Work out the finished part from the listing and answer in its coordinate system (mm). Coordinates: 2 decimals unless noted, no trailing zeros. Write each loop counter-clockwise with the first axis right and the second up, starting at its lowest first coordinate (ties: lowest second). Pieces come first, ordered by that corner, then holes. Notation, with made-up numbers: (9, -8.5) -> (13, -8.5) arc R4 ccw to (13, -2.5) -> close; hole circle Ø8 at (-34, 89.25). An arc over 180 degrees is marked (long way). Write each question's results on one line, items separated by ' | '. Start each with the question number.
Autodesk Inventor part; units mm, degrees
ref_plane "YZ Plane" through (0, 0, 0) normal (1, 0, 0) x (0, 1, 0)
ref_plane "XZ Plane" through (0, 0, 0) normal (0, 1, 0) x (-1, 0, 0)
ref_plane "XY Plane" through (0, 0, 0) normal (0, 0, 1) x (1, 0, 0)
sketch "スケッチ1" plane through (0, 0, 0) normal (0, 0, 1) x (1, 0, 0)
  circle A0 centre (0, 0) radius 8
  circle A1 centre (0, 0) radius 12
  dimension "d0" = 16
  dimension "d1" = 24
extrude "押し出し1" add sketch "スケッチ1" along normal blind 1
sketch "スケッチ2" plane through (0, 0, 1) normal (0, 0, 1) x (1, 0, 0)
  circle A0 centre (0, 0) radius 9
  circle A1 centre (0, 0) radius 12
  circle A2 centre (0, 0) radius 8
  dimension "d4" = 18
extrude "押し出し2" add sketch "スケッチ2" along normal blind 7 contours A0
chamfer "面取り1" distance 0.5 angle 45 1 edges at (-9, 0, 8)
properties part number "オイレスw10f16-18a" material "アセタール樹脂、黒"
1. Given pin 1 Ø1.5 at (x, z) = (5, 6.5) entering from -Y; pin 2 Ø3 at (y, z) = (-7.5, 6.5) entering from -X, each flat-ended and moving along its own axis, determine where each tip first touches the part or whether it passes through.
2. Find section A-A on x = 0. Give the vertices of the cut face in (y, z).
3. Find the intervals of material crossed by L1, parallel to Y at x = 0, z = 3.5; L2, parallel to Z at x = 1, y = -9.25; L3, parallel to Y at x = 3.25, z = 2.25, in increasing order.
4. Find section C-C on z = 2.5. Give the vertices of the cut face in (x, y).
5. Determine the mould class of faces 1 (the face through (2, 9, 1)), 2 (the face through (-1.73, 7.81, 3.94)), 3 (the face through (-1.172, -8.923, 4.204)) for opening direction Y: pulls with the +Y half, pulls with the -Y half, needs draft (parallel to the pull), parting line crosses it, or undercut.
Ans:
1) pin 1: stops at y = -7.93 | pin 2: stops at x = -6.71
2) outline: (-12, 0) -> (-8, 0) -> (-8, 8) -> (-8.5, 8) -> (-9, 7.5) -> (-9, 1) -> (-12, 1) -> close; (8, 0) -> (12, 0) -> (12, 1) -> (9, 1) -> (9, 7.5) -> (8.5, 8) -> (8, 8) -> close
3) L1: y = -9 to -8, 8 to 9 | L2: z = 0 to 1 | L3: y = -8.39 to -7.31, 7.31 to 8.39
4) outline: circle Ø18 at (0, 0); hole circle Ø16 at (0, 0)
5) face 1: needs draft | face 2: undercut | face 3: parting line crosses it
